Here's how the part is built. I have some questions about the finished solid (model axes, mm). A direction names the side the tool comes from. Coordinates: 2 decimals unless noted, no trailing zeros. Write each loop counter-clockwise with the first axis right and the second up, starting at its lowest first coordinate (ties: lowest second). Pieces come first, ordered by that corner, then holes.
```python
from build123d import *

# Parameters (mm, degrees)
F1_R     = 45
F2_R     = 30
F4_T     = -0.8
F5_R     = 7.5
F6_DEPTH = 10
F7_R     = 3.25
F8_DEPTH = 10.8010001
F9_R     = 3


with BuildPart() as f3:
    # F1 (on Top) → F3 section 0
    with BuildSketch(Plane.XY):
        Circle(F1_R)
    # F2 (on offset) → F3 section 1
    with BuildSketch(Plane.XY.offset(70)):
        Circle(F2_R)
    loft()

    # F4
    f4_openings = [f3.faces().sort_by_distance(p)[0] for p in [
        (0, 0, 0),
    ]]
    offset(amount=F4_T, openings=f4_openings, kind=Kind.INTERSECTION)

    # F5 (on face) → F6 (join)
    with BuildSketch(Plane(origin=(0, 0, 69.2), x_dir=(1, 0, 0), z_dir=(0, 0, -1))):
        Circle(F5_R)
    extrude(amount=F6_DEPTH)

    # F7 (on face) → F8 (cut, through all)
    with BuildSketch(Plane(origin=(0, 0, 59.2), x_dir=(1, 0, 0), z_dir=(0, 0, -1))):
        Circle(F7_R)
    extrude(amount=-F8_DEPTH, mode=Mode.SUBTRACT)

    # F9
    f9_edges = [f3.edges().sort_by_distance(p)[0] for p in [
        (-30, 0, 70),
    ]]
    fillet(f9_edges, radius=F9_R)


solid = f3.part
```
1) Will these pins go through, and if not, where does the flat tip stop? pin 1 (1 mm diameter, centred on y = -17.5, z = 57, fed in from -X); pin 2 (8 mm diameter, centred on y = 19.5, z = 35.5, fed in from -X); pin 3 (2 mm diameter, centred on x = -27.5, y = 13, fed in from +Z).
Values follow:
pin 1: stops at x = -28.06
pin 2: stops at x = -34.26
pin 3: stops at z = 69.37
2) We'd pull the mould along X, two halves only. Please class faces 3 (the face through (-27.788, -21.307, 42.773)), 4 (the face through (-28.602, -21.931, 41.802)), 5 (the face through (33, -30, 0)): pulls with the +X half, pulls with the -X half, needs draft (parallel to the pull), parting line crosses it, or undercut.
Values follow:
face 3: undercut
face 4: parting line crosses it
face 5: needs draft
3) On a 3-axis mill with a long thin cutter (end or side, diameter ignored), from which of +Z, -Z, +X, -X, +Y, -Y can I reach the whole of each face in a straight line? I mean faces 1 (the face through (-2.579, 1.978, 64.524)), 2 (the face through (-7.493, -0.33, 64.27)). Say none if no direction works.
Values follow:
face 1: +Z, -Z
face 2: -Z
4) Imagine slicing it at C-C on z = 18. Please give me the cut outline in (x, y).
Values follow:
outline: circle Ø82.29 at (0, 0); hole circle Ø80.65 at (0, 0)
5) Imagine slicing it at B-B on z = 10.5. Please give me the cut outline in (x, y).
Values follow:
outline: circle Ø85.5 at (0, 0); hole circle Ø83.86 at (0, 0)
6) Imagine slicing it at A-A on x = 0. Please give me the cut outline in (y, z), then the cut area to 3 significant figures.
Values follow:
outline: (-45, 0) - (-44.18, 0) - (-29.35, 69.2) - (-7.5, 69.2) - (-7.5, 59.2) - (-3.25, 59.2) - (-3.25, 70) - (-27.57, 70) arc R3 ccw to (-30.51, 67.63) - close; (3.25, 59.2) - (7.5, 59.2) - (7.5, 69.2) - (29.35, 69.2) - (44.18, 0) - (45, 0) - (30.51, 67.63) arc R3 ccw to (27.57, 70) - (3.25, 70) - close
area: 239 mm2
7) I need wall thicknesses on probe 1 along Y at (x, z) = (0, 64); probe 2 along Y at (x, z) = (0, 67); probe 3 along X at (y, z) = (0, 63.5). Which ranges of each line are inside material? Lowest first, please.
Values follow:
probe 1: y = -31.29 to -30.47, -7.5 to -3.25, 3.25 to 7.5, 30.47 to 31.29
probe 2: y = -30.64 to -29.82, -7.5 to -3.25, 3.25 to 7.5, 29.82 to 30.64
probe 3: x = -31.39 to -30.57, -7.5 to -3.25, 3.25 to 7.5, 30.57 to 31.39
